Geometry: see drawing. Coordinates: mm, zero at the bounding-box minimum. A direction names the side the tool comes from. Give positions to 0.01 mm unless a question says otherwise; leave off trailing zeros. Loops run counter-clockwise (first coordinate to the right, second up) from the corner with the lowest first, then second, coordinate; pieces in that order, holes last. Notation, with made-up numbers: (48.25, 20.5) -> (64.25, 20.5) arc R20 ccw to (64.25, 29.5) -> close; hole circle Ø6 at (62, -20.75). An arc over 180 degrees is marked (long way). Return JSON: item names as keys, results as strings. Group by question number.
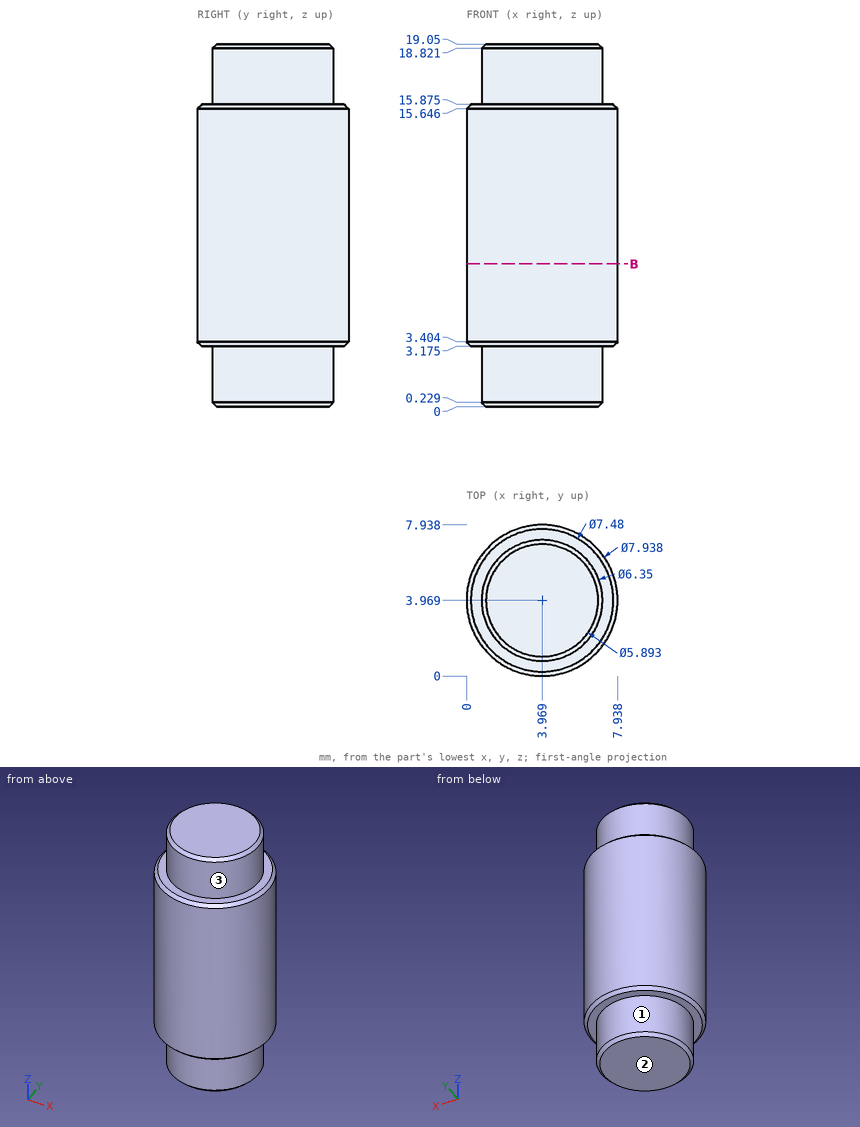
1) Material intervals for line 1 (Z direction, x = 7, y = 2) (1 decimal); line 2 (Y direction, x = 7.25, z = 14) (1 decimal); line 3 (X direction, y = 1.5, z = 10) (1 decimal), sorted ascending.
2) Contact query for flat-ended pins moving along their axis: P1, Ø1, axis at x = 2, z = 14, coming from the +Y side (1 decimal); P2, Ø3, axis at x = 7, z = 12, coming from the +Y side; P3, Ø2, axis at y = 6.5, z = 16.5, coming from the +X side. Output: stop coordinate, or through.
3) Reachability of the marked faces 1, 2 and 3 from +Z, -Z, +X, -X, +Y, -Y: full face, straight path, thin tool, end or side. Return the list, or none.
4) Cut plane B-B on z = 7.5. Return loops of the section in (x, y), then the cut area to 3 significant figures.
Calculated:
{
 "1": {"line 1": "3.2 to 15.9", "line 2": "1.7 to 6.2", "line 3": "0.9 to 7.1"},
 "2": {"P1": "y = 7.7", "P2": "y = 7.63", "P3": "x = 7.39"},
 "3": {"face 1": "-Z", "face 2": "-Z, +X, -X, +Y, -Y", "face 3": "+Z"},
 "4": {"outline": "circle Ø7.94 at (3.97, 3.97)", "area": "49.5 mm2"}
}
